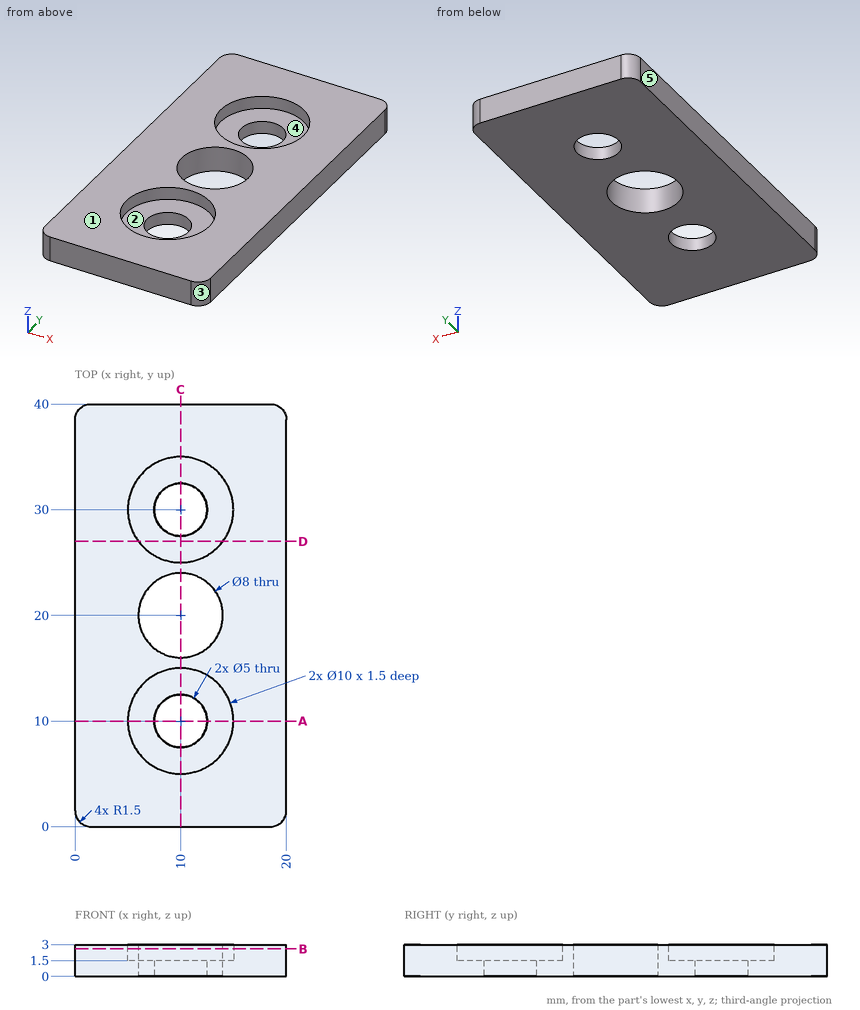
Check sheet for the drawn part. Datum: minimum x, y, z corner. Units: mm. A direction names the side the tool comes from. Give positions to 0.01 mm unless a question says otherwise; leave off trailing zeros. Order: outer loops, then holes, each group sorted by start corner. A loop starts at its lowest first (then second) coordinate and runs counter-clockwise, first axis right, second up. Notation, with made-up numbers: (-9.75, -21.75) - (49.25, -21.75) arc R25 cw to (49.25, 5.25) - close; hole circle Ø5 at (69.25, 54.5). An arc over 180 degrees is marked (long way). Answer in a Markdown table with one row per item. Add a question column.
Q1. Tool access check on the marked faces 4 and 5. Record the directions out of +Z, -Z, +X, -X, +Y, -Y that give a thin tool (end or side, any length) a straight path to the whole face; none if there is none.
Q2. Gauge pin test, flat end, axial feed: pin 1 (3 mm diameter, centred on x = 12, y = 31.5, fed in from +Z). Record the tip position at first contact, or that the pin passes through.
Q3. Mould release check, pull along X, two halves, no side actions. Record for the marked faces 1, 2 and 3: pulls with the +X half, pulls with the -X half, needs draft (parallel to the pull), parting line crosses it, or undercut.
Q4. Material ranges on probe 1 along Y at (x, z) = (10, 0.4); probe 2 along X at (y, z) = (10, 1.1); probe 3 along Z at (x, y) = (5.5, 31), recorded low to high. Write a range as from..to.
Q5. Cross-section at C-C, the plane x = 10. Enter the section's corners in (y, z).
Q6. Cross-section at D-D, the plane y = 27. Enter the section's corners in (x, z).
Q7. Cross-section at A-A, the plane y = 10. Enter the section's corners in (x, z).
Q8. Cross-section at B-B, the plane z = 2.6. Enter the section's corners in (x, y), then the cut area to 3 significant figures.
Check values:
| question | item | result |
|---|---|---|
| 1 | face 4 | +Z |
| 1 | face 5 | +Z, -Z, -X, +Y, -Y |
| 2 | pin 1 | stops at z = 1.5 |
| 3 | face 1 | needs draft |
| 3 | face 2 | undercut |
| 3 | face 3 | pulls with the +X half |
| 4 | probe 1 | y = 0..7.5, 12.5..16, 24..27.5, 32.5..40 |
| 4 | probe 2 | x = 0..7.5, 12.5..20 |
| 4 | probe 3 | z = 0..1.5 |
| 5 | outline | (0, 0) - (7.5, 0) - (7.5, 1.5) - (5, 1.5) - (5, 3) - (0, 3) - close; (12.5, 0) - (16, 0) - (16, 3) - (15, 3) - (15, 1.5) - (12.5, 1.5) - close; (24, 0) - (27.5, 0) - (27.5, 1.5) - (25, 1.5) - (25, 3) - (24, 3) - close; (32.5, 0) - (40, 0) - (40, 3) - (35, 3) - (35, 1.5) - (32.5, 1.5) - close |
| 6 | outline | (0, 0) - (20, 0) - (20, 3) - (14, 3) - (14, 1.5) - (6, 1.5) - (6, 3) - (0, 3) - close |
| 7 | outline | (0, 0) - (7.5, 0) - (7.5, 1.5) - (5, 1.5) - (5, 3) - (0, 3) - close; (12.5, 0) - (20, 0) - (20, 3) - (15, 3) - (15, 1.5) - (12.5, 1.5) - close |
| 8 | outline | (0, 1.5) arc R1.5 ccw to (1.5, 0) - (18.5, 0) arc R1.5 ccw to (20, 1.5) - (20, 38.5) arc R1.5 ccw to (18.5, 40) - (1.5, 40) arc R1.5 ccw to (0, 38.5) - close; hole circle Ø10 at (10, 10); hole circle Ø10 at (10, 30); hole circle Ø8 at (10, 20) |
| 8 | area | 591 mm^2 |
